Build history of the part. All positions in model axes, mm. Face numbers are marked on the shaded views. A direction names the side the tool comes from. Round coordinates to 2 decimals unless told otherwise and drop trailing zeros. Order: outer loops, then holes, each group sorted by start corner. A loop starts at its lowest first (then second) coordinate and runs counter-clockwise, first axis right, second up. Notation, with made-up numbers: (-11.5, 57.5) -> (-1.5, 57.5) arc R27 ccw to (-1.5, 85.5) -> close; hole circle Ø4 at (57, 74.25). An arc over 180 degrees is marked (long way). Write item = value, one per line.
from build123d import *

# Parameters (mm, degrees)
SKETCH1_W               = 50.8
SKETCH1_H               = 25.4
BOSS_EXTRUDE1_DEPTH     = 35.56
CUT_EXTRUDE1_DEPTH      = 51.545361805
CUT_EXTRUDE1_DEPTH_BACK = 51.545361805
SKETCH2_R               = 3.175
SKETCH2_W               = 25.4
SKETCH2_H               = 22.86
CUT_EXTRUDE2_DEPTH      = 64.296473835
CUT_EXTRUDE2_DEPTH_BACK = 64.296473835
SKETCH3_R               = 3.175
CHAMFER2_SIZE           = 6.35


with BuildPart() as part:
    # Sketch1 → Boss-Extrude1 (new body)
    with BuildSketch(Plane(origin=(0, 0, 0), x_dir=(1, 0, 0), z_dir=(0, 1, 0))):
        Rectangle(SKETCH1_W, SKETCH1_H)
    extrude(amount=BOSS_EXTRUDE1_DEPTH)

    # Sketch2 → Cut-Extrude1 (cut, two sides: drawn at the far end of the back side and taken through both)
    with BuildSketch(Plane.XY.offset(12.7).offset(-CUT_EXTRUDE1_DEPTH_BACK)):
        with Locations((0, 6.35)):
            Circle(SKETCH2_R)
        with Locations((0, 24.13)):
            Rectangle(SKETCH2_W, SKETCH2_H)
    extrude(amount=CUT_EXTRUDE1_DEPTH + CUT_EXTRUDE1_DEPTH_BACK, mode=Mode.SUBTRACT)

    # Sketch3 → Cut-Extrude2 (cut, two sides: drawn at the far end of the back side and taken through both)
    with BuildSketch(Plane(origin=(25.4, 0, 0), x_dir=(0, 0, -1), z_dir=(1, 0, 0)).offset(-CUT_EXTRUDE2_DEPTH_BACK)):
        with Locations(Location((0, 25.4, 0), (0, 0, 90))):
            Circle(SKETCH3_R)
    extrude(amount=CUT_EXTRUDE2_DEPTH + CUT_EXTRUDE2_DEPTH_BACK, mode=Mode.SUBTRACT)

    # Chamfer2
    chamfer2_edges = [part.edges().sort_by_distance(p)[0] for p in [
        (19.05, 35.56, -12.7),
        (19.05, 35.56, 12.7),
        (-19.05, 35.56, -12.7),
        (-19.05, 35.56, 12.7),
    ]]
    chamfer(chamfer2_edges, length=CHAMFER2_SIZE)


solid = part.part
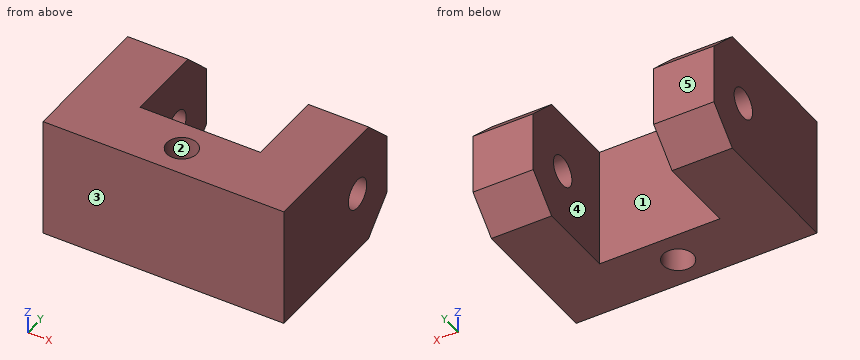
Q1. Cut at A-A, the plane y = 31. List the corners of the cut face in (x, z).
Check values:
outline = (-25.4, -10.91) -> (-12.7, -10.91) -> (-12.7, 10.91) -> (-25.4, 10.91) -> close; (12.7, -10.91) -> (25.4, -10.91) -> (25.4, 10.91) -> (12.7, 10.91) -> close
Q2. Probe probe 1 along X at (y, z) = (15.5, -7.25); probe 2 along Y at (x, z) = (19.75, 0) (3 decimals); probe 3 along X at (y, z) = (6.35, 7.5) (3 decimals). List the from-to ranges inside material, lowest first.
Check values:
probe_1 = -25.4 to -12.7, 12.7 to 25.4
probe_2 = 0 to 22.225, 28.575 to 35.56
probe_3 = -25.4 to -3.175, 3.175 to 25.4
Q3. Flat gauge pins, fed straight in: pin 1 (12 mm diameter, centred on x = -4.5, z = -2, fed in from +Y); pin 2 (1 mm diameter, centred on x = 12.5, y = 19.5, fed in from -Z). Where does each tip first touch, or does it go through?
Check values:
pin_1 = 12.7
pin_2 = -12.7
Q4. Mould opens along Y. For the marked faces 1, 2 and 3 say: released by +Y, released by -Y, zero draft, split by the parting line, or undercut.
Check values:
face_1 = released by +Y
face_2 = undercut
face_3 = released by -Y
Q5. Cut at B-B, the plane x = 0. List the corners of the cut face in (y, z) (3 decimals).
Check values:
outline = (0, -12.7) -> (3.175, -12.7) -> (3.175, 12.7) -> (0, 12.7) -> close; (9.525, -12.7) -> (12.7, -12.7) -> (12.7, 12.7) -> (9.525, 12.7) -> close
Q6. Which spindle directions (+Z, -Z, +X, -X, +Y, -Y) get a long thin tool onto all of the face, cutting with end or side? Do the marked faces 4 and 5. Say none if no direction does.
Check values:
face_4 = +Z, -Z, +Y
face_5 = +Z, -Z, +X, -X, +Y
Q7. Cut at C-C, the plane z = 1.75. List the corners of the cut face in (x, y) (3 decimals), and give its area (3 significant figures).
Check values:
outline = (-25.4, 0) -> (25.4, 0) -> (25.4, 22.751) -> (12.7, 22.751) -> (12.7, 12.7) -> (-12.7, 12.7) -> (-12.7, 22.751) -> (-25.4, 22.751) -> close; (-25.4, 28.049) -> (-12.7, 28.049) -> (-12.7, 35.56) -> (-25.4, 35.56) -> close; (12.7, 28.049) -> (25.4, 28.049) -> (25.4, 35.56) -> (12.7, 35.56) -> close; hole circle Ø6.35 at (0, 6.35)
area = 1,060 mm²
Q8. Cut at D-D, the plane y = 25.4. List the corners of the cut face in (x, z) (3 decimals), and give its area (3 significant figures).
Check values:
outline = (-25.4, -12.7) -> (-12.7, -12.7) -> (-12.7, -3.175) -> (-25.4, -3.175) -> close; (-25.4, 3.175) -> (-12.7, 3.175) -> (-12.7, 12.7) -> (-25.4, 12.7) -> close; (12.7, -12.7) -> (25.4, -12.7) -> (25.4, -3.175) -> (12.7, -3.175) -> close; (12.7, 3.175) -> (25.4, 3.175) -> (25.4, 12.7) -> (12.7, 12.7) -> close
area = 484 mm²
